from build123d import *

# Parameters (mm, degrees)
SKETCH1_W                                     = 3.5
SKETCH1_H                                     = 9.25
CBORE_FOR_0_SOCKET_HEAD_CAP_SCREW1_AT_2_COUNT = 2
CBORE_FOR_0_SOCKET_HEAD_CAP_SCREW1_AT_2_PITCH = 15.15867233
SKETCH5_OUTSIDE_W                             = 40.514
SKETCH5_OUTSIDE_H                             = 40.514
SKETCH5_OUTSIDE_W_2                           = 15.3924
SKETCH5_OUTSIDE_H_2                           = 15.3924
CUT_EXTRUDE1_DEPTH                            = 10
FILLET1_R                                     = 2.2606
SKETCH8_R                                     = 1.5
CUT_EXTRUDE2_DEPTH                            = 0.5
F_2_56_TAPPED_HOLE1_REACH                     = 22.332
F_2_56_TAPPED_HOLE1_BORE_R                    = 0.889


with BuildPart() as part:
    # Sketch1 → Revolve1 (revolve)
    with BuildSketch(Plane(origin=(0, 0, 0), x_dir=(0, 0, -1), z_dir=(1, 0, 0)), mode=Mode.PRIVATE) as revolve1_sk:
        with Locations((-1.75, 10.375)):
            Rectangle(SKETCH1_W, SKETCH1_H)
    revolve(revolve1_sk.sketch.rotate(Axis((0, 0, 0), (0, 0, -1)), 90), axis=Axis((0, 0, 0), (0, 0, -1)))  # turned: the seam where the file's is

    # Sketch3 → CBORE for #0 Socket Head Cap Screw1 (revolve, cut)
    with BuildSketch(Plane(origin=(5.359399999, 5.359399999, 3.5), x_dir=(0, -1, 0), z_dir=(1, 0, 0))):
        Polygon((0, 0), (0, 3.5), (1.44145, 3.5), (0.80645, 2.865), (0.80645, 1.524), (1.5875, 1.524), (1.5875, 0), align=None)
    cbore_for_0_socket_head_cap_screw1 = revolve(axis=Axis((5.359399999, 5.359399999, 9.85), (0, 0, -1)), mode=Mode.SUBTRACT)

    # CBORE for #0 Socket Head Cap Screw1 at 2: CBORE for #0 Socket Head Cap Screw1 ×2
    with Locations(*[Vector(-0.707106781, -0.707106781, 0) * (i * CBORE_FOR_0_SOCKET_HEAD_CAP_SCREW1_AT_2_PITCH) for i in range(1, CBORE_FOR_0_SOCKET_HEAD_CAP_SCREW1_AT_2_COUNT)]):
        add(cbore_for_0_socket_head_cap_screw1, mode=Mode.SUBTRACT)

    # Sketch5 outside → Cut-Extrude1 (cut)
    with BuildSketch(Plane.XY.offset(3.5)):
        Rectangle(SKETCH5_OUTSIDE_W, SKETCH5_OUTSIDE_H)
        Rectangle(SKETCH5_OUTSIDE_W_2, SKETCH5_OUTSIDE_H_2, mode=Mode.SUBTRACT)
    extrude(amount=-CUT_EXTRUDE1_DEPTH, mode=Mode.SUBTRACT)

    # Fillet1
    fillet1_edges = [part.edges().sort_by_distance(p)[0] for p in [
        (-7.6962, 7.6962, 1.75),
        (7.6962, 7.6962, 1.75),
        (7.6962, -7.6962, 1.75),
        (-7.6962, -7.6962, 1.75),
    ]]
    fillet(fillet1_edges, radius=FILLET1_R)

    # Sketch8 → Cut-Extrude2 (cut)
    with BuildSketch(Plane(origin=(-7.03408559, 7.03408559, 1.75), x_dir=(0, 0, 1), z_dir=(-0.707106781, 0.707106781, 0))):
        Circle(SKETCH8_R)
    extrude(amount=-CUT_EXTRUDE2_DEPTH, mode=Mode.SUBTRACT)

    # #2-56 Tapped Hole1 bore → #2-56 Tapped Hole1 (cut, up to next)
    with BuildSketch(Plane(origin=(-6.680532199, 6.680532199, 0), x_dir=(-0.707106781, -0.707106781, 0), z_dir=(-0.707106781, 0.707106781, 0)), mode=Mode.PRIVATE) as f_2_56_tapped_hole1_sk1:
        with Locations((0, 1.75)):
            Circle(F_2_56_TAPPED_HOLE1_BORE_R)
    f_2_56_tapped_hole1_tool1 = extrude(f_2_56_tapped_hole1_sk1.sketch, amount=-F_2_56_TAPPED_HOLE1_REACH, mode=Mode.PRIVATE) & part.part
    add(f_2_56_tapped_hole1_tool1.solids().sort_by_distance((-6.680532, 6.680532, 1.75))[0], mode=Mode.SUBTRACT)


solid = part.part
CAD build for the part. Positions are in the model's coordinates, mm. A direction names the side the tool comes from. Round coordinates to 2 decimals unless told otherwise and drop trailing zeros. Order: outer loops, then holes, each group sorted by start corner. A loop starts at its lowest first (then second) coordinate and runs counter-clockwise, first axis right, second up. Notation, with made-up numbers: M -40,43 L 10,43 A31 ccw 10,67 Z; hole C -13,44 d11. An arc over 180 degrees is marked long. Use one line per item in the form item = value.
Q1. Flat gauge pins, fed straight in: P1, Ø2, axis at x = -5.36, y = -5.36, coming from the +Z side; P2, Ø1.3, axis at x = 5.36, y = 5.36, coming from the -Z side; P3, Ø1.9, axis at x = 5.36, y = 5.36, coming from the -Z side. Where does each tip first touch, or does it go through?
Recorded:
P1 = 1.98
P2 = through
P3 = 0.49
Q2. Saw through at C-C on x = 5. State how many separate pieces and enclosed holes the cut face has, then the cut area to 3 significant figures.
Recorded:
separate_pieces = 3
enclosed_holes = 0
area = 26.0 mm^2
Q3. Probe L1, parallel to Y at x = 0, z = 1.2; L2, parallel to Y at x = 4.5, z = 3.35; L3, parallel to X at y = 4.25, z = 3.45. List the from-to ranges inside material, lowest first.
Recorded:
L1 = -7.7 to -5.75, 5.75 to 7.7
L2 = -7.7 to -3.58, 3.58 to 4.02, 6.69 to 7.7
L3 = -7.7 to -3.87, 3.87 to 4.22, 6.49 to 7.7
Q4. Which spindle directions (+Z, -Z, +X, -X, +Y, -Y) get a long thin tool onto all of the face, cutting with end or side? Do faces 1 (the cylindrical face through (7.02, 7.05, 1.73)), 2 (the cylindrical face through (-6.84, 6.8, 3.25)), 3 (the cylindrical face through (3.785, 5.566, 2.749)). Say none if no direction does.
Recorded:
face_1 = +Z, -Z, +X, +Y
face_2 = none
face_3 = +Z
Q5. Two-plate mould, pull along X, no slides. Class faces 4 (the flat face through (-7.696, 0, 2)), 5 (the cylindrical face through (-6.16, -5.25, 1.31)), 6 (the flat face through (5, -4, 0)): +X half, -X half, draft (parallel to the pull), parting line (faces both ways), or undercut.
Recorded:
face_4 = -X half
face_5 = undercut
face_6 = draft
Q6. Saw through at A-A on y = 0. Give the cut face in (x, z), then the cut area to 3 significant figures.
Recorded:
outline = M -7.7,0 L -5.75,0 L -5.75,3.5 L -7.7,3.5 Z; M 5.75,0 L 7.7,0 L 7.7,3.5 L 5.75,3.5 Z
area = 13.6 mm^2
